Can you work these out from the model? Positions are in its coordinate system, mm. Face numbers are marked on the shaded views. Coordinates: 2 decimals unless noted, no trailing zeros. Order: outer loops, then holes, each group sorted by start corner. A loop starts at its lowest first (then second) coordinate and runs counter-clockwise, first axis right, second up. Notation, with made-up numbers: (77.5, 63) - (127.5, 63) arc R22 cw to (127.5, 97) - close; hole circle Ø8 at (83, -12.75). An arc over 180 degrees is marked (long way). Return JSON: item names as keys, results as strings. Group by question number.
1) Imagine slicing it at A-A (z = 1.9). Write out the boundary of the cut face in (x, y), and give its area (3 significant figures).
2) If we mould it in two halves opening along Y, with no side actions, what happens to the marked faces 1, 2 and 3? For each: pulls with the +Y half, pulls with the -Y half, needs draft (parallel to the pull), parting line crosses it, or undercut.
3) Imagine slicing it at C-C (z = 0.5). Write out the boundary of the cut face in (x, y).
4) Imagine slicing it at B-B (y = -88). Write out the boundary of the cut face in (x, z).
5) For pin 1 Ø1.4 at (y, z) = (-100, 0.5) entering from -X; pin 2 Ø1 at (x, z) = (3.5, 0.5) entering from +Y; pin 3 Ø1 at (x, z) = (0, 0) entering from -Y, each with a flat end and sliding along its axis, tell me the tip position at first contact or that it passes through.
6) If I drill on line 1 along Y through (x, z) = (-1, 0.3); line 2 along Y through (x, z) = (2, -1.3); line 3 along X through (y, z) = (-99.25, -1), over which ranges is the centre line in solid material (lowest first)?
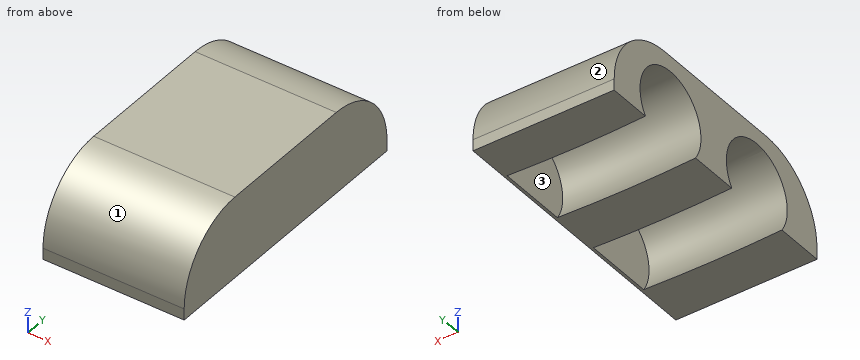
```python
from build123d import *

# Parameters (mm, degrees)
F5_W      = 10
F5_H      = 20
F6_DEPTH  = 5.8
F0_R      = 3
F2_R      = 3
F9_R      = 5
F11_DEPTH = 0.2


with BuildPart() as f6:
    # F5 (on offset) → F6 (new body)
    with BuildSketch(Plane.XY.offset(4.1)):
        with Locations((0, -95.8120375872)):
            Rectangle(F5_W, F5_H)
    extrude(amount=-F6_DEPTH)

    # F0 (on Front) → F7 (revolve, cut)
    with BuildSketch(Plane.XZ):
        with Locations((-91.5, 0)):
            Circle(F0_R)
    revolve(axis=Axis((0, 0, 0), (0, 0, 1)), mode=Mode.SUBTRACT)

    # F2 (on Front) → F8 (revolve, cut)
    with BuildSketch(Plane.XZ):
        with Locations((-100, 0)):
            Circle(F2_R)
    revolve(axis=Axis((0, 0, 0), (0, 0, 1)), mode=Mode.SUBTRACT)

    # F9
    f9_edges = [f6.edges().sort_by_distance(p)[0] for p in [
        (0, -105.812038, 4.1),
        (0, -85.812038, 4.1),
    ]]
    fillet(f9_edges, radius=F9_R)

    # F10 (on face) → F11 (join)
    with BuildSketch(Plane.YZ.offset(5)):
        with BuildLine():
            Line((-90.8120375872, 4.1), (-100.8120375872, 4.1))
            ThreePointArc((-100.8120375872, 4.1), (-104.3475714931, 2.6355339059), (-105.8120375872, -0.9))
            Line((-105.8120375872, -0.9), (-105.8120375872, -1.7))
            Line((-105.8120375872, -1.7), (-85.8120375872, -1.7))
            Line((-85.8120375872, -1.7), (-85.8120375872, -0.9))
            ThreePointArc((-85.8120375872, -0.9), (-87.2765036812, 2.6355339059), (-90.8120375872, 4.1))
        make_face()
    extrude(amount=-F11_DEPTH)


solid = f6.part
```
Calculated:
{
 "1": {"outline": "(-5, -104.95) - (5, -104.95) - (5, -86.67) - (-5, -86.67) - (-5, -89.04) arc R89.18 ccw to (4.8, -89.05) - (4.8, -93.7) arc R93.82 cw to (-5, -93.69) - (-5, -97.55) arc R97.68 ccw to (4.8, -97.56) - (4.8, -102.21) arc R102.32 cw to (-5, -102.2) - close", "area": "91.8 mm2"},
 "2": {"face 1": "pulls with the -Y half", "face 2": "pulls with the +Y half", "face 3": "undercut"},
 "3": {"outline": "(-5, -105.61) - (5, -105.61) - (5, -86.01) - (-5, -86.01) - (-5, -88.4) arc R88.54 ccw to (4.8, -88.41) - (4.8, -94.34) arc R94.46 cw to (-5, -94.33) - (-5, -96.91) arc R97.04 ccw to (4.8, -96.92) - (4.8, -102.85) arc R102.96 cw to (-5, -102.84) - close"},
 "4": {"outline": "(-5, -1.7) - (5, -1.7) - (5, 3.23) - (-5, 3.23) - close"},
 "5": {"pin 1": "x = 4.8", "pin 2": "y = -85.89", "pin 3": "y = -105.8"},
 "6": {"line 1": "-105.67 to -102.98, -97.01 to -94.48, -88.51 to -85.96", "line 2": "-105.81 to -102.68, -97.28 to -94.18, -88.77 to -85.81", "line 3": "4.8 to 5"}
}
